```python
from build123d import *

# Parameters (mm, degrees)
SKETCH1_R           = 2.032
SKETCH1_R_2         = 14.351
SKETCH1_W           = 25.4
SKETCH1_H           = 76.2
BOSS_EXTRUDE1_DEPTH = 3.175
SKETCH2_R           = 2.032
CUT_EXTRUDE1_DEPTH  = 69.759094853
SKETCH4_W           = 3.175
SKETCH4_H           = 25.4
BOSS_EXTRUDE2_DEPTH = 38.1
SKETCH5_R           = 2.032
CUT_EXTRUDE2_DEPTH  = 69.759094853
FILLET5_R           = 2.54
SKETCH6_W           = 46.838855708
SKETCH6_H           = 19.05
BOSS_EXTRUDE3_DEPTH = 3.175
SKETCH7_R           = 2.032
CUT_EXTRUDE3_DEPTH  = 75.018388912
FILLET6_R           = 2.54


with BuildPart() as part:
    # Sketch1 → Boss-Extrude1 (new body)
    # profile 1 of 2: a face of its own
    with BuildSketch(Plane.XY):
        Polygon((-57.15, -19.108999882), (-12.7, -19.108999882), (-12.7, 24.638), (-12.7, 27.881000118), (-57.15, 27.881000118), align=None)
        with Locations((-52.832, -14.790999882)):
            Circle(SKETCH1_R, mode=Mode.SUBTRACT)
        with Locations((-17.018, -14.790999882)):
            Circle(SKETCH1_R, mode=Mode.SUBTRACT)
        with Locations((-34.925, 4.386000118)):
            Circle(SKETCH1_R_2, mode=Mode.SUBTRACT)
    # profile 2 of 2: a face of its own
    with BuildSketch(Plane.XY):
        Rectangle(SKETCH1_W, SKETCH1_H)
    extrude(amount=BOSS_EXTRUDE1_DEPTH)

    # Sketch2 → Cut-Extrude1 (cut, through all)
    with BuildSketch(Plane.XY.offset(3.175)):
        Circle(SKETCH2_R)
        with Locations((0, 12.7)):
            Circle(SKETCH2_R)
        with Locations((0, 25.4)):
            Circle(SKETCH2_R)
        with Locations((0, -12.7)):
            Circle(SKETCH2_R)
        with Locations((0, -25.4)):
            Circle(SKETCH2_R)
    extrude(amount=-CUT_EXTRUDE1_DEPTH, mode=Mode.SUBTRACT)

    # Sketch4 → Boss-Extrude2 (add)
    with BuildSketch(Plane(origin=(12.7, 0, 0), x_dir=(0, 0, -1), z_dir=(1, 0, 0))):
        with Locations((-1.5875, -25.4)):
            Rectangle(SKETCH4_W, SKETCH4_H)
    extrude(amount=BOSS_EXTRUDE2_DEPTH)

    # Sketch5 → Cut-Extrude2 (cut, through all)
    with BuildSketch(Plane(origin=(0, 0, 0), x_dir=(-1, 0, 0), z_dir=(0, 0, -1))):
        with Locations(Location((0, -25.4, 0), (0, 0, 180))):
            Circle(SKETCH5_R)
        with Locations((-12.7, -25.4)):
            Circle(SKETCH5_R)
        with Locations((-25.4, -25.4)):
            Circle(SKETCH5_R)
        with Locations((-38.1, -25.4)):
            Circle(SKETCH5_R)
    extrude(amount=-CUT_EXTRUDE2_DEPTH, mode=Mode.SUBTRACT)

    # Fillet5
    fillet5_edges = [part.edges().sort_by_distance(p)[0] for p in [
        (12.7, 38.1, 1.5875),
        (-12.7, -38.1, 1.5875),
        (-57.15, -19.108999882, 1.5875),
        (12.7, -12.7, 1.5875),
        (50.8, -38.1, 1.5875),
        (50.8, -12.7, 1.5875),
    ]]
    fillet(fillet5_edges, radius=FILLET5_R)

    # Sketch6 → Boss-Extrude3 (add)
    with BuildSketch(Plane(origin=(0, 0, 0), x_dir=(-1, 0, 0), z_dir=(0, 0, -1))):
        with Locations((33.730572146, 37.406000118)):
            Rectangle(SKETCH6_W, SKETCH6_H)
    extrude(amount=-BOSS_EXTRUDE3_DEPTH)

    # Sketch7 → Cut-Extrude3 (cut, through all)
    with BuildSketch(Plane(origin=(0, 0, 0), x_dir=(-1, 0, 0), z_dir=(0, 0, -1))):
        with Locations((25.4, 36.771000118)):
            Circle(SKETCH7_R)
        with Locations((38.1, 36.771000118)):
            Circle(SKETCH7_R)
        with Locations((50.8, 36.771000118)):
            Circle(SKETCH7_R)
    extrude(amount=-CUT_EXTRUDE3_DEPTH, mode=Mode.SUBTRACT)

    # Fillet6
    fillet6_edges = [part.edges().sort_by_distance(p)[0] for p in [
        (-10.311144292, 46.931000118, 1.5875),
        (-57.15, 46.931000118, 1.5875),
    ]]
    fillet(fillet6_edges, radius=FILLET6_R)


solid = part.part
```
Geometry check sheet. Reference: the model listing, model coordinates, mm. A direction names the side the tool comes from. Round coordinates to 2 decimals unless told otherwise and drop trailing zeros. Loops run counter-clockwise (first coordinate to the right, second up) from the corner with the lowest first, then second, coordinate; pieces in that order, holes last. Notation, with made-up numbers: (-33.75, 49.5) - (19.25, 49.5) arc R16 cw to (19.25, 65.5) - close; hole circle Ø7 at (81.25, -22). An arc over 180 degrees is marked (long way). Write item = value, one per line. Start each with the question number.
1. Set-up check for faces 1 (the face through (0, 38.1, 2)), 2 (the face through (-34, -19.109, 2)), 3 (the face through (-4, 4, 0)): record each of +Z, -Z, +X, -X, +Y, -Y from which the full face is reachable in a straight line by a thin tool's end or side.
2. Section check B-B on x = 38.1. Enter the section's corners in (y, z) (3 decimals).
3. Mould release check, pull along X, two halves, no side actions. Record for faces 4 (the face through (-0.44, 23.416, 1.61)), 5 (the face through (19, -38.1, 2)), 6 (the face through (-10.311, 41, 2)): released by +X, released by -X, zero draft, split by the parting line, or undercut.
4. Thickness scan on line 1 (Y direction, x = 0, z = 1.85); line 2 (X direction, y = 12, z = 2.2); line 3 (X direction, y = -34, z = 0.4). Record the ranges inside material, lowest first.
5. Section check A-A on y = 25.4. Enter the section's corners in (x, z) (3 decimals), then the cut area to 3 significant figures.
6. Section check D-D on z = 1. Give the number of separate pieces and of enclosed holes in the cut face, then the cut area to 3 significant figures.
7. Depth check by flat-ended pin: pin 1 (1.5 mm diameter, centred on x = 8, y = 28.5, fed in from -Z); pin 2 (1 mm diameter, centred on y = 41, z = 1, fed in from +X); pin 3 (1 mm diameter, centred on x = -36.5, z = 1.5, fed in from -Y); pin 4 (1.6 mm diameter, centred on x = 4.5, z = 1.5, fed in from +Y). Enter the tip coordinate at first touch or a pass-through.
8. Section check C-C on y = -25.4. Enter the section's corners in (x, z) (3 decimals), then the cut area to 3 significant figures.
Working result:
q1.face_1 = +Z, -Z, +X, +Y
q1.face_2 = +Z, -Z, -X, -Y
q1.face_3 = -Z, +X, -X, +Y, -Y
q2.outline = (-38.1, 0) - (-27.432, 0) - (-27.432, 3.175) - (-38.1, 3.175) - close; (-23.368, 0) - (-12.7, 0) - (-12.7, 3.175) - (-23.368, 3.175) - close
q3.face_4 = undercut
q3.face_5 = zero draft
q3.face_6 = released by +X
q4.line_1 = -38.1 to -27.43, -23.37 to -14.73, -10.67 to -2.03, 2.03 to 10.67, 14.73 to 23.37, 27.43 to 38.1
q4.line_2 = -57.15 to -47.09, -22.76 to -1.91, 1.91 to 12.7
q4.line_3 = -12.7 to 50.8
q5.outline = (-57.15, 0) - (-2.032, 0) - (-2.032, 3.175) - (-57.15, 3.175) - close; (2.032, 0) - (12.7, 0) - (12.7, 3.175) - (2.032, 3.175) - close
q5.area = 209 mm^2
q6.separate_pieces = 1
q6.enclosed_holes = 14
q6.area = 5,040 mm^2
q7.pin_1 = 0
q7.pin_2 = -10.31
q7.pin_3 = -19.11
q7.pin_4 = 38.1
q8.outline = (-12.7, 0) - (-2.032, 0) - (-2.032, 3.175) - (-12.7, 3.175) - close; (2.032, 0) - (10.668, 0) - (10.668, 3.175) - (2.032, 3.175) - close; (14.732, 0) - (23.368, 0) - (23.368, 3.175) - (14.732, 3.175) - close; (27.432, 0) - (36.068, 0) - (36.068, 3.175) - (27.432, 3.175) - close; (40.132, 0) - (50.8, 0) - (50.8, 3.175) - (40.132, 3.175) - close
q8.area = 150 mm^2
